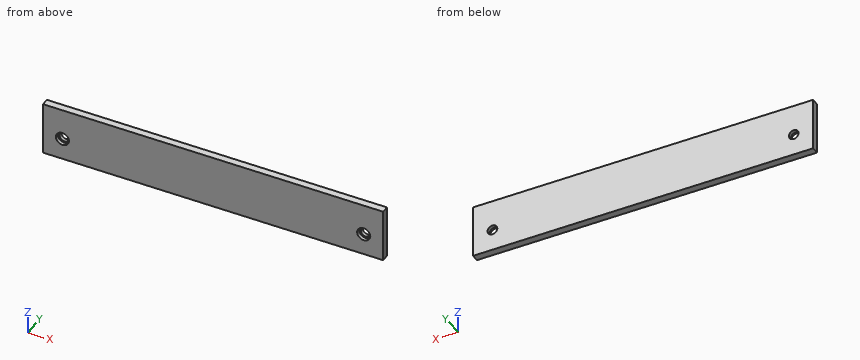
```python
from build123d import *

# Parameters (mm, degrees)
F0_W     = 19.05
F0_H     = 139.7
F1_DEPTH = 444.5
F2_R     = 12.7
F3_DEPTH = 19.051
F4_R     = 17.145
F4_R_2   = 12.7
F5_DEPTH = 9.525


with BuildPart() as f1:
    # F0 (on Right) → F1 (new body, symmetric)
    with BuildSketch(Plane.YZ):
        Rectangle(F0_W, F0_H)
    extrude(amount=F1_DEPTH, both=True)

    # F2 (on face) → F3 (cut, through all)
    with BuildSketch(Plane.XZ.offset(9.525)):
        with Locations((-393.7, -12.7)):
            Circle(F2_R)
        with Locations((393.7, -12.7)):
            Circle(F2_R)
    extrude(amount=-F3_DEPTH, mode=Mode.SUBTRACT)

    # F4 (on face) → F5 (cut)
    with BuildSketch(Plane.XZ.offset(9.525)):
        with Locations((-393.7, -12.7)):
            Circle(F4_R)
        with Locations((-393.7, -12.7)):
            Circle(F4_R_2, mode=Mode.SUBTRACT)
        with Locations((393.7, -12.7)):
            Circle(F4_R)
        with Locations((393.7, -12.7)):
            Circle(F4_R_2, mode=Mode.SUBTRACT)
        with Locations((-393.7, -12.7)):
            Circle(F4_R_2)
    extrude(amount=-F5_DEPTH, mode=Mode.SUBTRACT)


solid = f1.part
```
Build history of the part. All positions in model axes, mm. Give positions to 0.01 mm unless a question says otherwise; leave off trailing zeros. Order: outer loops, then holes, each group sorted by start corner. A loop starts at its lowest first (then second) coordinate and runs counter-clockwise, first axis right, second up. Notation, with made-up numbers: M 75.5,-6 L 127.5,-6 A22 ccw 127.5,7 Z; hole C 7,10.5 d6. An arc over 180 degrees is marked long. Return JSON: item names as keys, results as strings.
Q1. Wall check: probe 1 along Z at (x, y) = (394.5, 8); probe 2 along X at (y, z) = (3.5, -5.5); probe 3 along Z at (x, y) = (-393.7, -2.5) (3 decimals). Give the ranges that are in metal, low to high. Write a range as from..to.
Answer list:
{"probe 1": "z = -69.85..-25.37, -0.03..69.85", "probe 2": "x = -444.5..-404.16, -383.24..383.24, 404.16..444.5", "probe 3": "z = -69.85..-29.845, 4.445..69.85"}
Q2. Flat gauge pins, fed straight in: pin 1 (23 mm diameter, centred on x = -393.7, z = -12.7, fed in from -Y); pin 2 (17 mm diameter, centred on x = 400.5, z = -7.5, fed in from -Y). Where does each tip first touch, or does it go through?
Answer list:
{"pin 1": "passes through", "pin 2": "stops at y = 0"}
Q3. Band-saw the part on B-B (z = -12.7). Give the cut face in (x, y) (3 decimals).
Answer list:
{"outline": "M -444.5,-9.525 L -410.845,-9.525 L -410.845,0 L -406.4,0 L -406.4,9.525 L -444.5,9.525 Z; M -381,0 L -376.555,0 L -376.555,-9.525 L 376.555,-9.525 L 376.555,0 L 381,0 L 381,9.525 L -381,9.525 Z; M 406.4,0 L 410.845,0 L 410.845,-9.525 L 444.5,-9.525 L 444.5,9.525 L 406.4,9.525 Z"}
Q4. Band-saw the part on A-A (x = -393.7). Give the cut face in (y, z) (3 decimals).
Answer list:
{"outline": "M -9.525,-69.85 L 9.525,-69.85 L 9.525,-25.4 L 0,-25.4 L 0,-29.845 L -9.525,-29.845 Z; M -9.525,4.445 L 0,4.445 L 0,0 L 9.525,0 L 9.525,69.85 L -9.525,69.85 Z"}
